Source: CAD feature listing. Evaluate the final solid. Frame: model axes, mm. Coordinates: 2 decimals unless noted, no trailing zeros. Order: outer loops, then holes, each group sorted by start corner. A loop starts at its lowest first (then second) coordinate and runs counter-clockwise, first axis right, second up. Notation, with made-up numbers: (5.25, 68.25) -> (55.25, 68.25) arc R6 ccw to (55.25, 74.25) -> close; hole circle Ø2 at (35.5, -32.5). An arc over 180 degrees is marked (long way). Put each result on its own line as item: value.
from build123d import *

# Parameters (mm, degrees)
SKETCH1_W           = 200
SKETCH1_H           = 12
BOSS_EXTRUDE1_DEPTH = 12
SKETCH3_W           = 12
SKETCH3_H           = 75
CUT_EXTRUDE1_DEPTH  = 12


with BuildPart() as part:
    # Sketch1 → Boss-Extrude1 (new body)
    with BuildSketch(Plane(origin=(0, 0, 0), x_dir=(1, 0, 0), z_dir=(0, 1, 0))):
        Polygon((200, 75), (-200, 75), (-200, -75), (-100, -75), (-100, -63), (100, -63), (100, -75), (200, -75), align=None)
        with Locations((0, -81)):
            Rectangle(SKETCH1_W, SKETCH1_H)
        with Locations((0, -69)):
            Rectangle(SKETCH1_W, SKETCH1_H)
    extrude(amount=BOSS_EXTRUDE1_DEPTH)

    # Sketch3 → Cut-Extrude1 (cut)
    with BuildSketch(Plane(origin=(0, 12, 0), x_dir=(1, 0, 0), z_dir=(0, 1, 0))):
        with Locations((-144, 0)):
            Rectangle(SKETCH3_W, SKETCH3_H)
    cut_extrude1 = extrude(amount=-CUT_EXTRUDE1_DEPTH, mode=Mode.SUBTRACT)

    # Mirror1: Cut-Extrude1 across plane
    add(cut_extrude1.mirror(Plane(origin=(0, 0, 0), x_dir=(0, 0, 1), z_dir=(1, 0, 0))), mode=Mode.SUBTRACT)


solid = part.part
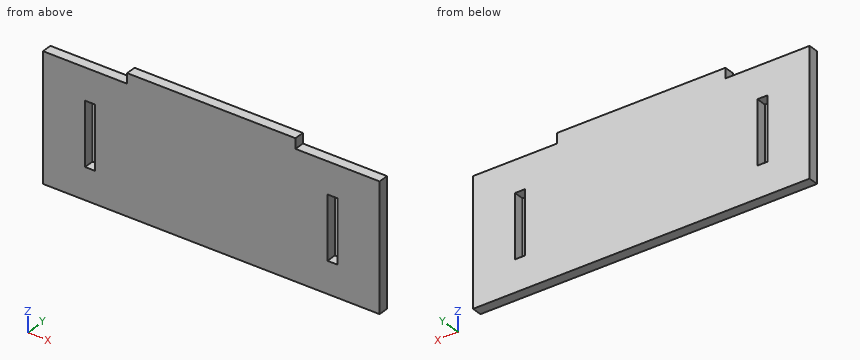
1. Cut plane A-A on z = -5. Output: boundary loops of the cut face in (x, y).
Numbers:
outline: (-200, 0) -> (-150, 0) -> (-150, 12) -> (-200, 12) -> close; (-138, 0) -> (138, 0) -> (138, 12) -> (-138, 12) -> close; (150, 0) -> (200, 0) -> (200, 12) -> (150, 12) -> close
2. Cut plane C-C on x = 128. Output: boundary loops of the cut face in (y, z), plus the area to 3 significant figures.
Numbers:
outline: (0, -75) -> (12, -75) -> (12, 75) -> (0, 75) -> close
area: 1,800 mm2
3. Ray query, line 1 along X through (y, z) = (3.5, -32.5); line 2 along Z through (x, y) = (127.5, 3.5). Return the intervals inside material, ascending.
Numbers:
line 1: x = -200 to -150, -138 to 138, 150 to 200
line 2: z = -75 to 75
4. First-contact query: pin 1 (3.5 mm diameter, centred on y = 8, z = 78.5, fed in from +X). Flat tip, straight axial feed; report the tip coordinate or a pass-through.
Numbers:
pin 1: stops at x = 100
5. Cut plane B-B on y = 8.75. Output: boundary loops of the cut face in (x, z), plus the area to 3 significant figures.
Numbers:
outline: (-200, -75) -> (200, -75) -> (200, 75) -> (100, 75) -> (100, 87) -> (-100, 87) -> (-100, 75) -> (-200, 75) -> close; hole (-150, -37.5) -> (-138, -37.5) -> (-138, 37.5) -> (-150, 37.5) -> close; hole (138, -37.5) -> (150, -37.5) -> (150, 37.5) -> (138, 37.5) -> close
area: 60,600 mm2
